The figure shows three views and two pictorial views of one solid part (mm, origin at its lowest corner). Answer the questions. Give positions to 0.01 mm unless a question says otherwise; leave off trailing zeros. Loops run counter-clockwise (first coordinate to the right, second up) from the corner with the lowest first, then second, coordinate; pieces in that order, holes last. Notation, with made-up numbers: (77.5, 78) - (101.5, 78) arc R18 ccw to (101.5, 104) - close; hole circle Ø8 at (61, 84.5). An arc over 180 degrees is marked (long way). One line per question, with ' | ' between items.
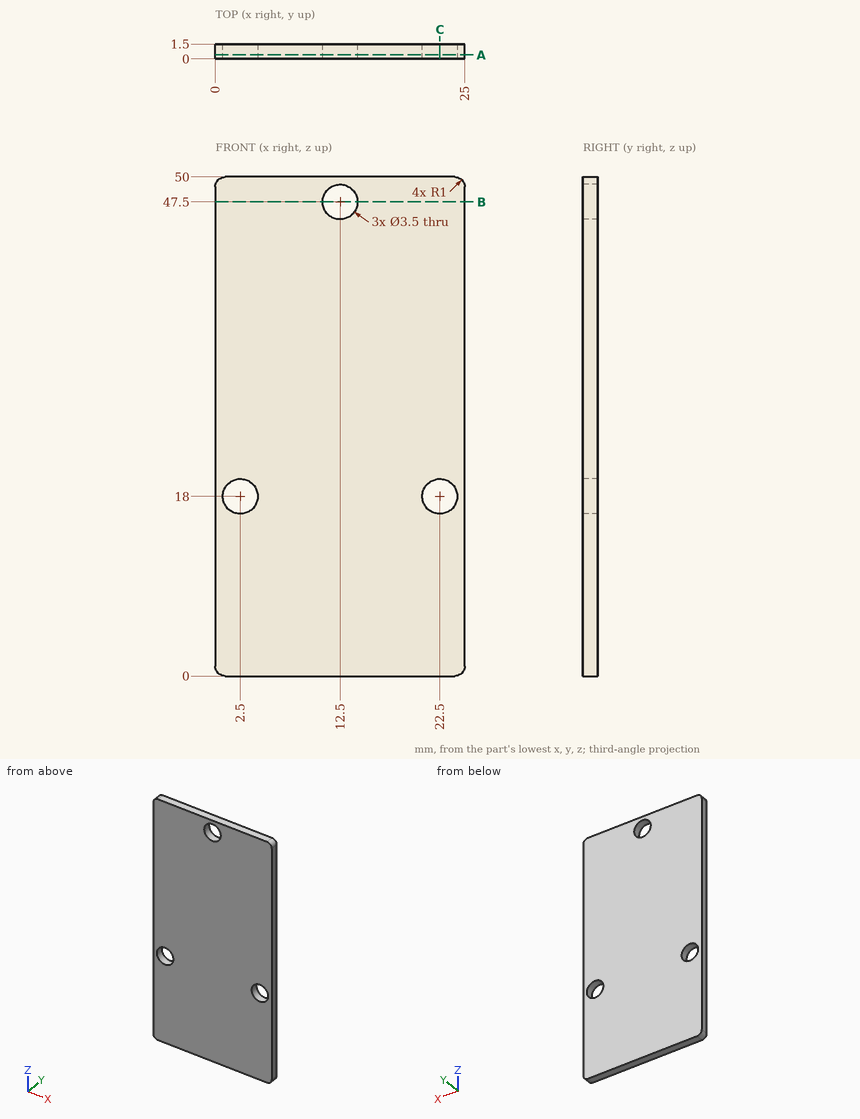
1. Find section A-A on y = 0.4. Write down the section's boundary in (x, z).
Evaluation:
outline: (0, 1) arc R1 ccw to (1, 0) - (24, 0) arc R1 ccw to (25, 1) - (25, 49) arc R1 ccw to (24, 50) - (1, 50) arc R1 ccw to (0, 49) - close; hole circle Ø3.5 at (2.5, 18); hole circle Ø3.5 at (12.5, 47.5); hole circle Ø3.5 at (22.5, 18)
2. Find section C-C on x = 22.5. Write down the section's boundary in (y, z).
Evaluation:
outline: (0, 0) - (1.5, 0) - (1.5, 16.25) - (0, 16.25) - close; (0, 19.75) - (1.5, 19.75) - (1.5, 50) - (0, 50) - close
3. A flat-ended cylindrical pin translates along its axis: pin 1 (4 mm diameter, centred on x = 12.5, z = 47.5, fed in from -Y). Find the tip coordinate at first contact, or state that the pin passes through.
Evaluation:
pin 1: y = 0
4. Consider L1, parallel to Z at x = 12.5, y = 1; L2, parallel to Z at x = 22.5, y = 0.55; L3, parallel to X at y = 0.3, z = 19. Determine where each line is inside the solid, lowest interval first.
Evaluation:
L1: 0 to 45.75, 49.25 to 50 | L2: 0 to 16.25, 19.75 to 50 | L3: 0 to 1.06, 3.94 to 21.06, 23.94 to 25
5. Find section B-B on z = 47.5. Write down the section's boundary in (x, y), then the cut area to 4 significant figures.
Evaluation:
outline: (0, 0) - (10.75, 0) - (10.75, 1.5) - (0, 1.5) - close; (14.25, 0) - (25, 0) - (25, 1.5) - (14.25, 1.5) - close | area: 32.25 mm2
